Autodesk Inventor part; units mm, degrees
ref_plane "YZ Plane" through (0, 0, 0) normal (1, 0, 0) x (0, 1, 0)
ref_plane "XZ Plane" through (0, 0, 0) normal (0, 1, 0) x (-1, 0, 0)
ref_plane "XY Plane" through (0, 0, 0) normal (0, 0, 1) x (1, 0, 0)
sketch "Sketch1" plane through (0, 0, 0) normal (0, 1, 0) x (-1, 0, 0)
  circle A0 centre (0, 0) radius 27.94
  dimension "d0" = 55.88
extrude "Extrusion1" add sketch "Sketch1" along normal blind 5.08
sketch "Sketch2" plane through (0, 5.08, 0) normal (0, 1, 0) x (1, 0, 0)
  circle A0 centre (0, 0) radius 13.97
  dimension "d3" = 27.94
extrude "Extrusion2" add sketch "Sketch2" along normal blind 5.842
sketch "Sketch3" plane through (0, 10.922, 0) normal (0, 1, 0) x (1, 0, 0)
  circle A0 centre (0, 0) radius 11.811
  dimension "d6" = 23.622
extrude "Extrusion3" add sketch "Sketch3" along normal blind 10.16
sketch "Sketch5" plane through (0, 21.082, 0) normal (0, 1, 0) x (1, 0, 0)
  line L0 (0, 0) -> (0, 2.667)
  line L1 (-3.1168, 0) -> (-1.5584, 2.6992)
  line L2 (-1.5584, 2.6992) -> (1.5584, 2.6992)
  line L3 (1.5584, 2.6992) -> (3.1168, 0)
  line L4 (3.1168, 0) -> (1.5584, -2.6992)
  line L5 (1.5584, -2.6992) -> (-1.5584, -2.6992)
  line L6 (-1.5584, -2.6992) -> (-3.1168, 0)
  dimension "d10" = 2.667
extrude "Extrusion4" cut sketch "Sketch5" against normal blind 25.4
sketch "Sketch6" plane through (0, 5.08, 0) normal (0, 1, 0) x (1, 0, 0)
  circle A0 centre (0, 0) radius 27.94
  line L0 (0, -27.94) -> (0, -26.162)
  line L1 (0, -26.162) -> (0, -24.257)
  circle A1 centre (0, -24.257) radius 1.905
  dimension "d13" = 1.778
  dimension "d14" = 1.905
extrude "Extrusion5" cut sketch "Sketch6" against normal blind 25.4 contours A1
sketch "Sketch7" plane through (0, 21.082, 0) normal (0, 1, 0) x (1, 0, 0)
  point P0 (0, 0)
  point P1 (0, 0)
pattern_circular "Circular Pattern1" count 6 over 360 about axis through (0, 21.082, 0) along (0, 1, 0) of "Extrusion5"
properties part number "Wheel Mount"
Could you check a few things on this model? Use its own coordinates, in mm. A direction names the side the tool comes from. Coordinates: 2 decimals unless noted, no trailing zeros. Order: outer loops, then holes, each group sorted by start corner. A loop starts at its lowest first (then second) coordinate and runs counter-clockwise, first axis right, second up. Notation, with made-up numbers: (-1, -21) - (45, -21) arc R18 cw to (45, 13) - close; hole circle Ø5 at (53, 59). An arc over 180 degrees is marked (long way). Answer in a Markdown table with one row per item. Add a question column.
(1) If we mould it in two halves opening along X, with no side actions, what happens to faces 4 (the face through (-9.37, 15.93, -7.19)), 5 (the face through (2.35, 10.69, 1.33)), 6 (the face through (-19.104, 2.576, 12.212)), 7 (the face through (-6, 5.08, 13))? For each: released by +X, released by -X, zero draft, split by the parting line, or undercut.
(2) If we section it at A-A, the plane x = 0: Please give me the cut outline in (y, z).
(3) On a 3-axis mill with a long thin cutter (end or side, diameter ignored), from which of +Z, -Z, +X, -X, +Y, -Y can I reach the whole of each face in a straight line? I mean faces 1 (the face through (-2.327, 10.689, 1.368)), 2 (the face through (-6, 0, 0)), 3 (the face through (-1.82, 7.96, 13.85)). Say none if no direction works.
(4) I need wall thicknesses on L1, parallel to Z at x = 0, y = 2.8; L2, parallel to Y at x = -14.5, z = 14.5; L3, parallel to Y at x = 5.5, z = -10.5. Which ranges of each line are inside material? Lowest first, please.
(5) If we section it at B-B, the plane y = 15.5: Please give me the cut outline in (x, z).
(6) Will these pins go through, and if not, where does the flat tip stop? pin 1 (2 mm diameter, centred on x = 12, z = -7.5, fed in from +Y); pin 2 (4 mm diameter, centred on y = 7.5, z = 9, fed in from +X); pin 3 (0.9 mm diameter, centred on x = 0.5, y = 9.5, fed in from +Z).
(7) If we section it at D-D, the plane z = 12.5: Please give me the cut outline in (x, y).
(8) If we section it at C-C, the plane z = 23.5: Please give me the cut outline in (x, y), then the cut area to 3 significant figures.
Results are:
| question | item | result |
|---|---|---|
| 1 | face 4 | split by the parting line |
| 1 | face 5 | undercut |
| 1 | face 6 | undercut |
| 1 | face 7 | zero draft |
| 2 | outline | (0, -27.94) - (5.08, -27.94) - (5.08, -26.16) - (0, -26.16) - close; (0, -22.35) - (5.08, -22.35) - (5.08, -13.97) - (10.92, -13.97) - (10.92, -11.81) - (21.08, -11.81) - (21.08, -2.7) - (0, -2.7) - close; (0, 2.7) - (21.08, 2.7) - (21.08, 11.81) - (10.92, 11.81) - (10.92, 13.97) - (5.08, 13.97) - (5.08, 22.35) - (0, 22.35) - close; (0, 26.16) - (5.08, 26.16) - (5.08, 27.94) - (0, 27.94) - close |
| 3 | face 1 | +Y, -Y |
| 3 | face 2 | +Z, -Z, +X, -X, -Y |
| 3 | face 3 | +Y |
| 4 | L1 | z = -27.94 to -26.16, -22.35 to -2.7, 2.7 to 22.35, 26.16 to 27.94 |
| 4 | L2 | y = 0 to 5.08 |
| 4 | L3 | y = 0 to 10.92 |
| 5 | outline | circle Ø23.62 at (0, 0); hole (-3.12, 0) - (-1.56, -2.7) - (1.56, -2.7) - (3.12, 0) - (1.56, 2.7) - (-1.56, 2.7) - close |
| 6 | pin 1 | stops at y = 10.92 |
| 6 | pin 2 | stops at x = 12.09 |
| 6 | pin 3 | stops at z = 13.97 |
| 7 | outline | (-24.99, 0) - (-22.88, 0) - (-22.88, 5.08) - (-24.99, 5.08) - close; (-19.14, 0) - (19.14, 0) - (19.14, 5.08) - (6.24, 5.08) - (6.24, 10.92) - (-6.24, 10.92) - (-6.24, 5.08) - (-19.14, 5.08) - close; (22.88, 0) - (24.99, 0) - (24.99, 5.08) - (22.88, 5.08) - close |
| 8 | outline | (-15.11, 0) - (-1.75, 0) - (-1.75, 5.08) - (-15.11, 5.08) - close; (1.75, 0) - (15.11, 0) - (15.11, 5.08) - (1.75, 5.08) - close |
| 8 | area | 136 mm2 |
